The listing builds one solid part. Answer for the finished solid, in the listing's coordinates (mm). Give positions to 0.01 mm unless a question says otherwise; leave off trailing zeros. Write each question's results on one line, items separated by ' | '. Start each with the question number.
Autodesk Inventor part; units mm, degrees
ref_plane "YZ Plane" through (0, 0, 0) normal (1, 0, 0) x (0, 1, 0)
ref_plane "XZ Plane" through (0, 0, 0) normal (0, 1, 0) x (-1, 0, 0)
ref_plane "XY Plane" through (0, 0, 0) normal (0, 0, 1) x (1, 0, 0)
ref_plane "Piano di lavoro1" through (-9.854, -197.5144, 1.4226) normal (0, 0, -1) x (1, 0, 0)
sketch "Schizzo1" plane through (-9.854, -197.5144, 1.4226) normal (0, 0, -1) x (1, 0, 0)
  line L0 (302.439, 120.7317) -> (292.439, 120.7317)
  line L1 (292.439, 120.7317) -> (292.439, -79.2683)
  line L2 (292.439, -79.2683) -> (302.439, -79.2683)
  line L3 (302.439, -79.2683) -> (302.439, 120.7317)
  point P0 (9.854, -197.5144)
  dimension "d0" = 200
  dimension "d1" = 10
extrude "Estrusione1" add sketch "Schizzo1" along normal blind 200
sketch "Schizzo2" plane through (292.585, -318.2462, 1.4226) normal (1, 0, 0) x (0, 0, -1)
  circle A0 centre (180, 100) radius 11
  line L0 (0, 0) -> (200, 0)
  line L1 (200, 0) -> (200, 200)
  line L2 (200, 200) -> (0, 200)
  line L3 (0, 200) -> (0, 0)
  circle A1 centre (164.5, 84.5) radius 1.75
  circle A2 centre (164.5, 115.5) radius 1.75
  circle A3 centre (195.5, 115.5) radius 1.75
  circle A4 centre (195.5, 84.5) radius 1.75
  point P0 (200, 100)
  dimension "d4" = 22
  dimension "d5" = 200
  dimension "d6" = 200
  dimension "d7" = 100
  dimension "d9" = 31
  dimension "d10" = 31
  dimension "d11" = 15.5
  dimension "d12" = 31
  dimension "d13" = 31
  dimension "d14" = 0
  dimension "d15" = 15.5
  dimension "d16" = 0
  dimension "d17" = 3.5
  dimension "d18" = 3.5
  dimension "d19" = 3.5
  dimension "d20" = 3.5
  dimension "d22" = 20
extrude "Estrusione2" cut sketch "Schizzo2" against normal blind 10 contours A0 | A1 | A2 | A3 | A4
equation "\"d10\" = d9"
equation "\"d11\" = 0.5 * d9"
equation "\"d12\" = d9"
equation "\"d13\" = d9"
equation "\"d15\" = 0.5 * d9"
equation "\"d18\" = d17"
equation "\"d19\" = d17"
equation "\"d20\" = d17"
properties part number "piano z"
1. This flat-tipped pin is pushed along its axis until it touches: pin 1 Ø3 at (y, z) = (-202.75, -194.08) entering from -X. Where does it stop, or does it pass through?
2. Consider probe 1 along Y at (x, z) = (287, -176.5); probe 2 along Z at (x, y) = (287, -202); probe 3 along Y at (x, z) = (286.25, -170). Determine where each line is inside the solid, lowest interval first. Write a range as [from, to].
3. The mould has two halves that part along Y. Classify faces 1 (the cylindrical face through (287.65, -217.76, -167.59)), 2 (the flat face through (282.585, -220, -97)), 3 (the flat face through (288, -318.246, -97)): pulls with the +Y half, pulls with the -Y half, needs draft (parallel to the pull), parting line crosses it, or undercut.
Results:
1) pin 1: passes through
2) probe 1: y = [-318.25, -229.05], [-207.44, -118.25] | probe 2: z = [-198.58, -195.66], [-192.49, -164.66], [-161.49, 1.42] | probe 3: y = [-318.25, -225.13], [-211.36, -118.25]
3) face 1: undercut | face 2: needs draft | face 3: pulls with the -Y half
